from build123d import *

# Parameters (mm, degrees)
SKETCH_R          = 70
SKETCH_R_2        = 68
PAD_DEPTH         = 2
CYLINDER001_R     = 2
CYLINDER001_DEPTH = 4
ARRAY001_COUNT    = 14
CYLINDER_R        = 3
CYLINDER_DEPTH    = 4
ARRAY_COUNT       = 4
SKETCH002_R       = 70
PAD001_DEPTH      = 2


with BuildPart() as body:
    # Sketch → Pad (new body)
    with BuildSketch(Plane.XY):
        Circle(SKETCH_R)
        Circle(SKETCH_R_2, mode=Mode.SUBTRACT)
    extrude(amount=PAD_DEPTH)


with BuildPart() as array001:
    # Cylinder001 → Cylinder001 (new body)
    with BuildSketch(Plane(origin=(64, 0, -3), x_dir=(1, 0, 0), z_dir=(0, 0, 1))):
        Circle(CYLINDER001_R)
    extrude(amount=CYLINDER001_DEPTH)

    # Array001: Array001 ×14 about axis
    array001_axis = Axis((0, 0, 0), (0, 0, 1))


with BuildPart() as array001_1:
    add(array001.part)
    for i in range(1, ARRAY001_COUNT):
        add(array001.part.rotate(array001_axis, i * 360 / ARRAY001_COUNT))


with BuildPart() as array:
    # Cylinder → Cylinder (new body)
    with BuildSketch(Plane(origin=(11, 0, 0), x_dir=(1, 0, 0), z_dir=(0, 0, 1))):
        Circle(CYLINDER_R)
    extrude(amount=CYLINDER_DEPTH)

    # Array: Array ×4 about axis
    array_axis = Axis((0, 0, 0), (0, 0, 1))


with BuildPart() as array_1:
    add(array.part)
    for i in range(1, ARRAY_COUNT):
        add(array.part.rotate(array_axis, i * 360 / ARRAY_COUNT))


with BuildPart() as array_2:
    # Array placement: moved
    add(array_1.part.moved(Location((0, 0, -3))))


with BuildPart() as fusion:
    # Sketch002 → Pad001 (new body)
    with BuildSketch(Plane.XY):
        Circle(SKETCH002_R)
    extrude(amount=PAD001_DEPTH)


with BuildPart() as fusion_1:
    # Body001 placement: moved
    add(fusion.part.moved(Location((0, 0, -2))))

    # Cut: cut Array
    add(array_2.part, mode=Mode.SUBTRACT)

    # Cut001: cut Array001
    add(array001_1.part, mode=Mode.SUBTRACT)

    # Fusion: union Body
    add(body.part)


solid = fusion_1.part
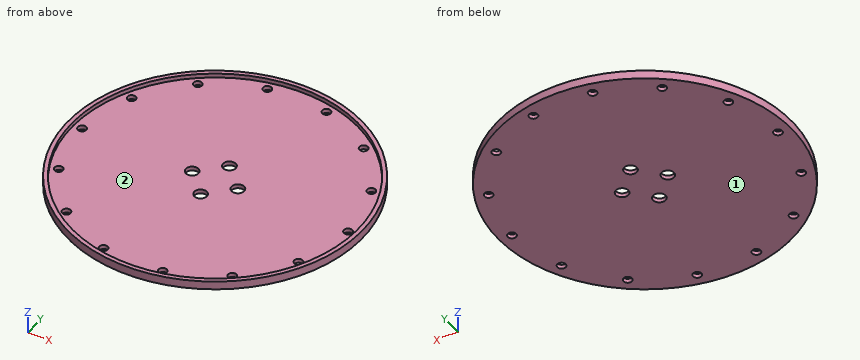
Geometry: final body of the model. Coordinates: model frame, mm. Face numbers are marked on the shaded views. Coordinates: 2 decimals unless noted, no trailing zeros. Order: outer loops, then holes, each group sorted by start corner. A loop starts at its lowest first (then second) coordinate and runs counter-clockwise, first axis right, second up. Notation, with made-up numbers: (-24.5, 13) - (-13.5, 13) arc R23 ccw to (-13.5, 40) - close; hole circle Ø8 at (-18.5, -36). An arc over 180 degrees is marked (long way). Use one line per item in the form item = value.
1) Mould query, pull axis Y, two halves, no side actions, for the marked faces 1 and 2. Classes: +Y half, -Y half, draft (parallel to the pull), parting line (faces both ways), or undercut.
Solutions:
face_1 = draft
face_2 = undercut
2) Section C-C (x = -64). Return loops of the section in (y, z), then the cut area to 3 significant figures.
Solutions:
outline = (-28.35, -2) - (-2, -2) - (-2, 0) - (-22.98, 0) - (-22.98, 2) - (-28.35, 2) - close; (2, -2) - (28.35, -2) - (28.35, 2) - (22.98, 2) - (22.98, 0) - (2, 0) - close
area = 127 mm^2
3) Section D-D (y = -54). Return loops of the section in (x, z), then the cut area to 3 significant figures.
Solutions:
outline = (-44.54, -2) - (44.54, -2) - (44.54, 2) - (41.33, 2) - (41.33, 0) - (-41.33, 0) - (-41.33, 2) - (-44.54, 2) - close
area = 191 mm^2
4) Pin query (flat end, axial travel): pin 1 (2.5 mm diameter, centred on x = -14.24, y = 62.4, fed in from -Z); pin 2 (4.5 mm diameter, centred on x = 14.24, y = -62.4, fed in from -Z); pin 3 (1.5 mm diameter, centred on x = -25, y = -29, fed in from +Z); pin 4 (1 mm diameter, centred on y = -49, z = -1, fed in from -X). Return the tip coordinate at first contact, or that it passes through.
Solutions:
pin_1 = through
pin_2 = -2
pin_3 = 0
pin_4 = -50.48
5) Ray query, L1, parallel to X at y = 2, z = 0.6; L2, parallel to Z at x = -35, y = 0.5; L3, parallel to Y at x = -17, z = 0.7. Return the intervals inside material, ascending.
Solutions:
L1 = -69.97 to -67.97, 67.97 to 69.97
L2 = -2 to 0
L3 = -67.9 to -65.84, 65.84 to 67.9
6) Section B-B (x = 0). Return loops of the section in (y, z).
Solutions:
outline = (-70, -2) - (-14, -2) - (-14, 0) - (-68, 0) - (-68, 2) - (-70, 2) - close; (-8, -2) - (8, -2) - (8, 0) - (-8, 0) - close; (14, -2) - (70, -2) - (70, 2) - (68, 2) - (68, 0) - (14, 0) - close
7) Section A-A (y = 0). Return loops of the section in (x, z).
Solutions:
outline = (-70, -2) - (-66, -2) - (-66, 0) - (-68, 0) - (-68, 2) - (-70, 2) - close; (-62, -2) - (-14, -2) - (-14, 0) - (-62, 0) - close; (-8, -2) - (8, -2) - (8, 0) - (-8, 0) - close; (14, -2) - (62, -2) - (62, 0) - (14, 0) - close; (66, -2) - (70, -2) - (70, 2) - (68, 2) - (68, 0) - (66, 0) - close
